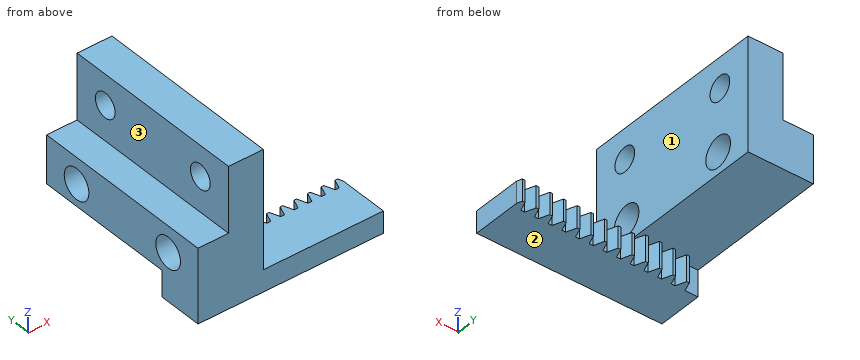
```python
from build123d import *

# Parameters (mm, degrees)
BLANKSKE_W                 = 40
BLANKSKE_H                 = 12.5
BLANK_DEPTH                = 5
TOOTHCUTSIM_DEPTH          = 43.20485754
TEETHCUTS_COUNT            = 14
TEETHCUTS_PITCH            = 3.14159265
MOVE_FACE1_BY              = 0.44
SKETCH1_W                  = 15
SKETCH1_H                  = 43
BOSS_EXTRUDE1_DEPTH        = 12
F_7_0_7_DIAMETER_HOLE1_D   = 7
SKETCH6_W                  = 2.7
SKETCH6_H                  = 17
BOSS_EXTRUDE2_DEPTH        = 3.5
SKETCH7_W                  = 8
SKETCH7_H                  = 43
BOSS_EXTRUDE3_DEPTH        = 15
F_5_6_5_6_DIAMETER_HOLE1_D = 5.6
CUT_EXTRUDE1_START         = -17
SKETCH11_W                 = 15
SKETCH11_H                 = 3.5
CUT_EXTRUDE1_DEPTH         = 17
MOVE_FACE2_BY              = 1
MOVE_FACE3_BY              = 3


with BuildPart() as part:
    # BlankSke → Blank (new body)
    with BuildSketch(Plane.XY):
        with Locations((20, 6.25)):
            Rectangle(BLANKSKE_W, BLANKSKE_H)
    extrude(amount=-BLANK_DEPTH)

    # TooCutSkeSim → ToothCutSim (cut, through all)
    with BuildSketch(Plane.XY):
        Polygon((0.44443537, 10.25), (-0.44443537, 10.25), (-1.272613241, 12.5254), (1.272613241, 12.5254), align=None)
    toothcutsim = extrude(amount=-TOOTHCUTSIM_DEPTH, mode=Mode.SUBTRACT)

    # TeethCuts: ToothCutSim ×14
    with Locations(*[(i * TEETHCUTS_PITCH, 0, 0) for i in range(1, TEETHCUTS_COUNT)]):
        add(toothcutsim, mode=Mode.SUBTRACT)

    # Move Face1: a face moved inward by 0.44
    extrude(part.faces().sort_by_distance((0, 5.125, -2.5))[0], amount=MOVE_FACE1_BY, dir=(1, 0, 0), mode=Mode.SUBTRACT)

    # Sketch1 → Boss-Extrude1 (add)
    with BuildSketch(Plane(origin=(0, 0, 0), x_dir=(-1, 0, 0), z_dir=(0, 0, -1))):
        with Locations((-4.94, 21.5)):
            Rectangle(SKETCH1_W, SKETCH1_H)
    extrude(amount=-BOSS_EXTRUDE1_DEPTH)

    # Ø7.0 (7) Diameter Hole1 (through all)
    with Locations(Plane.ZY.offset(2.56)):
        with Locations((6, 34.5), (6, 8.5)):
            Hole(F_7_0_7_DIAMETER_HOLE1_D / 2)

    # Sketch6 → Boss-Extrude2 (add)
    with BuildSketch(Plane.XZ):
        with Locations((-1.21, 3.5)):
            Rectangle(SKETCH6_W, SKETCH6_H)
        with Locations((11.09, 3.5)):
            Rectangle(SKETCH6_W, SKETCH6_H)
    extrude(amount=BOSS_EXTRUDE2_DEPTH)

    # Sketch7 → Boss-Extrude3 (add)
    with BuildSketch(Plane.XY.offset(12)):
        with Locations((8.44, 21.5)):
            Rectangle(SKETCH7_W, SKETCH7_H)
    extrude(amount=BOSS_EXTRUDE3_DEPTH)

    # Ø5.6 (5.6) Diameter Hole1 (through all)
    with Locations(Plane(origin=(12.44, 0, 0), x_dir=(0, 0, -1), z_dir=(1, 0, 0))):
        with Locations((-20, 35), (-20, 8)):
            Hole(F_5_6_5_6_DIAMETER_HOLE1_D / 2)

    # Sketch11 → Cut-Extrude1 (cut)
    with BuildSketch(Plane.XY.offset(12).offset(CUT_EXTRUDE1_START)):
        with Locations((4.94, -1.75)):
            Rectangle(SKETCH11_W, SKETCH11_H)
    extrude(amount=CUT_EXTRUDE1_DEPTH, mode=Mode.SUBTRACT)

    # Move Face2: a face moved inward by 1.0
    extrude(part.faces().sort_by_distance((4.543546999, 25.718346506, 0))[0], amount=MOVE_FACE2_BY, dir=(0, 0, 1), mode=Mode.SUBTRACT)

    # Move Face3: a face moved outward by 3.0
    extrude(part.faces().sort_by_distance((0.44, 5.125, -2))[0], amount=MOVE_FACE3_BY, dir=(-1, 0, 0))


solid = part.part
```
Source: CAD feature listing. Evaluate the final solid. Frame: model axes, mm. Face numbers are marked on the shaded views. A direction names the side the tool comes from. Coordinates: 2 decimals unless noted, no trailing zeros. Write each loop counter-clockwise with the first axis right and the second up, starting at its lowest first coordinate (ties: lowest second). Pieces come first, ordered by that corner, then holes. Notation, with made-up numbers: (59, 70.25) -> (88, 70.25) arc R31 cw to (88, 103.25) -> close; hole circle Ø4 at (13, 86.25). An arc over 180 degrees is marked (long way). Return JSON: item names as keys, results as strings. Group by question number.
1) Section query B-B, the plane y = 19. Return loops of the section in (x, z), plus the area to 3 significant figures.
2) Set-up query: the marked faces 1, 2 and 3. Return all of +Z, -Z, +X, -X, +Y, -Y with unobstructed straight access to the full face (end or side cutting, diameter ignored); none if empty.
3) Section query A-A, the plane z = 20. Return loops of the section in (x, y), plus the area to 3 significant figures.
4) Ray query, line 1 along Y through (x, z) = (8, 20); line 2 along Y through (x, z) = (2.75, 6); line 3 along Z through (x, y) = (4, 26.5). Return the intervals inside material, ascending.
5) Contact query for flat-ended pins moving along their axis: P1, Ø6, axis at x = 32, y = 4, coming from the +Z side; P2, Ø0.5, axis at x = 36.5, z = -3.5, coming from the +Y side; P3, Ø7.5, axis at x = 2.5, y = 32, coming from the -Z side. Output: stop coordinate, or through.
6) Section query C-C, the plane z = 6. Return loops of the section in (x, y).
From the geometry:
{
 "1": {"outline": "(-2.56, 1) -> (12.44, 1) -> (12.44, 27) -> (4.44, 27) -> (4.44, 12) -> (-2.56, 12) -> close", "area": "285 mm²"},
 "2": {"face 1": "+Z, +X, +Y, -Y", "face 2": "-Z, +X, -X, +Y, -Y", "face 3": "+Z, -X, +Y, -Y"},
 "3": {"outline": "(4.44, 0) -> (12.44, 0) -> (12.44, 5.2) -> (4.44, 5.2) -> close; (4.44, 10.8) -> (12.44, 10.8) -> (12.44, 32.2) -> (4.44, 32.2) -> close; (4.44, 37.8) -> (12.44, 37.8) -> (12.44, 43) -> (4.44, 43) -> close", "area": "254 mm²"},
 "4": {"line 1": "0 to 5.2, 10.8 to 32.2, 37.8 to 43", "line 2": "0 to 5, 12 to 31, 38 to 43", "line 3": "1 to 12"},
 "5": {"P1": "z = 0", "P2": "y = 12.5", "P3": "z = 1"},
 "6": {"outline": "(-2.56, 0) -> (12.44, 0) -> (12.44, 5) -> (-2.56, 5) -> close; (-2.56, 12) -> (12.44, 12) -> (12.44, 31) -> (-2.56, 31) -> close; (-2.56, 38) -> (12.44, 38) -> (12.44, 43) -> (-2.56, 43) -> close"}
}
